Could you check a few things on this drawing? It's one solid part, dimensions in mm from its lowest x, y, z. A direction names the side the tool comes from. Give positions to 0.01 mm unless a question says otherwise; leave off trailing zeros. Order: outer loops, then holes, each group sorted by start corner. A loop starts at its lowest first (then second) coordinate and runs counter-clockwise, first axis right, second up. Notation, with made-up numbers: (47, 89) -> (68, 89) arc R16 ccw to (68, 109) -> close; hole circle Ø11 at (-40, 74). An arc over 180 degrees is marked (long way). Answer as a JSON object with one key per item and string values.
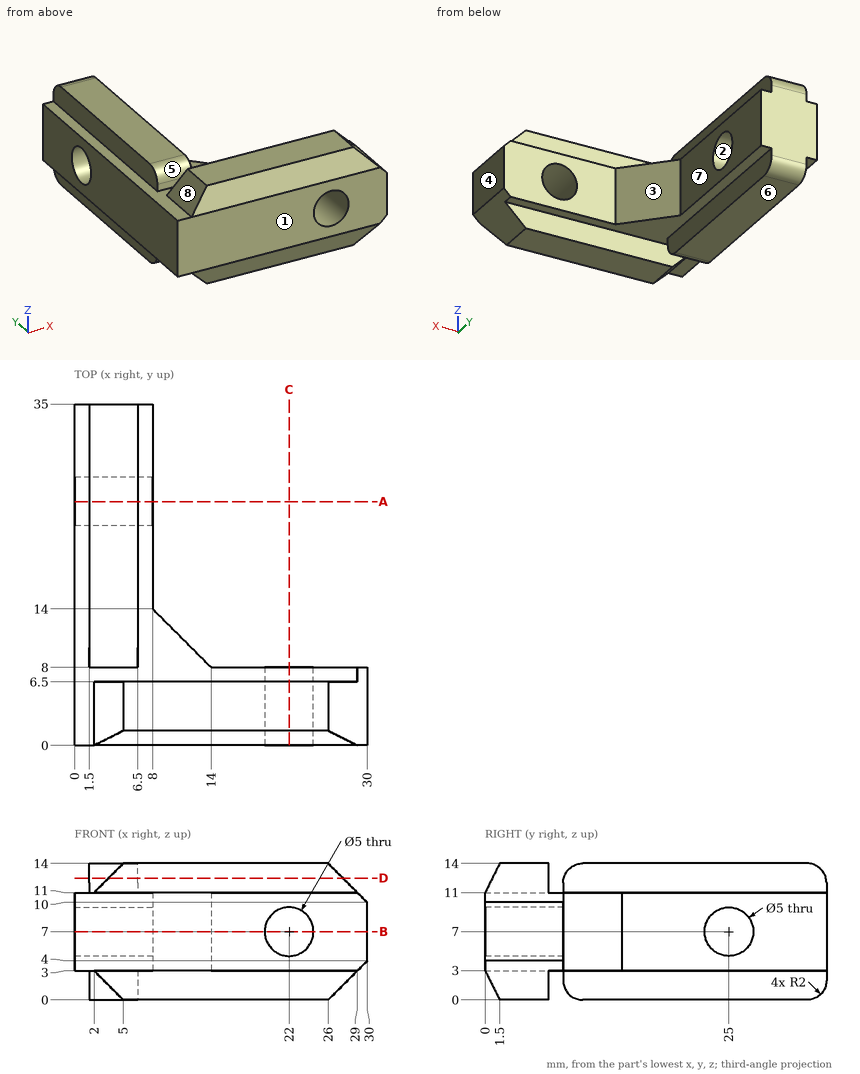
1. If we section it at D-D on z = 12.5: Please give me the cut outline in (x, y).
Worked answers:
{"outline": "(1.5, 8.06) -> (6.5, 8.06) -> (6.5, 34.94) -> (1.5, 34.94) -> close; (3.5, 0.75) -> (27.5, 0.75) -> (27.5, 6.5) -> (3.5, 6.5) -> close"}
2. If we section it at C-C on x = 22: Please give me the cut outline in (y, z).
Worked answers:
{"outline": "(0, 3) -> (1.5, 0) -> (6.5, 0) -> (6.5, 3) -> (8, 3) -> (8, 4.5) -> (0, 4.5) -> close; (0, 9.5) -> (8, 9.5) -> (8, 11) -> (6.5, 11) -> (6.5, 14) -> (1.5, 14) -> (0, 11) -> close"}
3. If we mould it in two halves opening along Y, with no side actions, what happens to the marked faces 1, 2, 3 and 4? For each: +Y half, -Y half, draft (parallel to the pull), parting line (faces both ways), or undercut.
Worked answers:
{"face 1": "-Y half", "face 2": "undercut", "face 3": "+Y half", "face 4": "draft"}
4. Please list where these lines run through material, in increasing order: L1, parallel to Y at x = 5, z = 7; L2, parallel to Z at x = 22, y = 5.5; L3, parallel to X at y = 19, z = 7.5.
Worked answers:
{"L1": "0 to 22.5, 27.5 to 35", "L2": "0 to 4.5, 9.5 to 14", "L3": "0 to 8"}
5. If we section it at B-B on z = 7: Please give me the cut outline in (x, y), then the cut area to 3 significant figures.
Worked answers:
{"outline": "(0, 0) -> (19.5, 0) -> (19.5, 8) -> (14, 8) -> (8, 14) -> (8, 22.5) -> (0, 22.5) -> close; (0, 27.5) -> (8, 27.5) -> (8, 35) -> (0, 35) -> close; (24.5, 0) -> (30, 0) -> (30, 8) -> (24.5, 8) -> close", "area": "394 mm²"}
6. For the marked faces 5, 6, 7 and 8, which set-ups out of +Z, -Z, +X, -X, +Y, -Y let a thin tool reach every point of the face, with its end or its side?
Worked answers:
{"face 5": "+Z, +X, -X", "face 6": "-Z, +X, -X, +Y, -Y", "face 7": "+Z, -Z, +X, +Y", "face 8": "+Z, -X, -Y"}
7. Will these pins go through, and if not, where does the flat tip stop? pin 1 Ø4 at (y, z) = (25, 7) entering from +X; pin 2 Ø6 at (x, z) = (23.5, 2.5) entering from +Y; pin 3 Ø2.5 at (y, z) = (29.5, 8) entering from +X; pin 4 Ø1.5 at (y, z) = (26.5, 1) entering from -X.
Worked answers:
{"pin 1": "through", "pin 2": "y = 8", "pin 3": "x = 8", "pin 4": "x = 1.5"}
8. If we section it at A-A on y = 25: Please give me the cut outline in (x, z).
Worked answers:
{"outline": "(0, 3) -> (1.5, 3) -> (1.5, 0) -> (6.5, 0) -> (6.5, 3) -> (8, 3) -> (8, 4.5) -> (0, 4.5) -> close; (0, 9.5) -> (8, 9.5) -> (8, 11) -> (6.5, 11) -> (6.5, 14) -> (1.5, 14) -> (1.5, 11) -> (0, 11) -> close"}
